```python
from build123d import *

# Parameters (mm, degrees)
F0_R     = 1.55
F1_DEPTH = 4
F2_R     = 3
F3_DEPTH = 3


with BuildPart() as f1:
    # F0 (on Top) → F1 (new body)
    with BuildSketch(Plane.XY):
        Polygon((25.166199, 37.371666), (-19.243801, 37.371666), (-19.243801, -14.908334), (-24.348801, -14.908334), (-24.348801, -32.808334), (30.271199, -32.808334), (30.271199, -6.428334), (25.166199, -6.428334), align=None)
        with Locations((-20.908801, -17.408334)):
            Circle(F0_R, mode=Mode.SUBTRACT)
        with Locations((27.351199, -18.678334)):
            Circle(F0_R, mode=Mode.SUBTRACT)
        with Locations((-6.183801, 33.401666)):
            Circle(F0_R, mode=Mode.SUBTRACT)
        with Locations((21.756199, 33.401666)):
            Circle(F0_R, mode=Mode.SUBTRACT)
    extrude(amount=F1_DEPTH)

    # F2 (on face) → F3 (cut)
    with BuildSketch(Plane.XY.offset(4)):
        with Locations((-20.908801, -17.408334)):
            Circle(F2_R)
        with Locations((27.452319, -18.754228)):
            Circle(F2_R)
        with Locations((-6.183801, 33.401666)):
            Circle(F2_R)
        with Locations((21.756199, 33.401666)):
            Circle(F2_R)
    extrude(amount=-F3_DEPTH, mode=Mode.SUBTRACT)


solid = f1.part
```
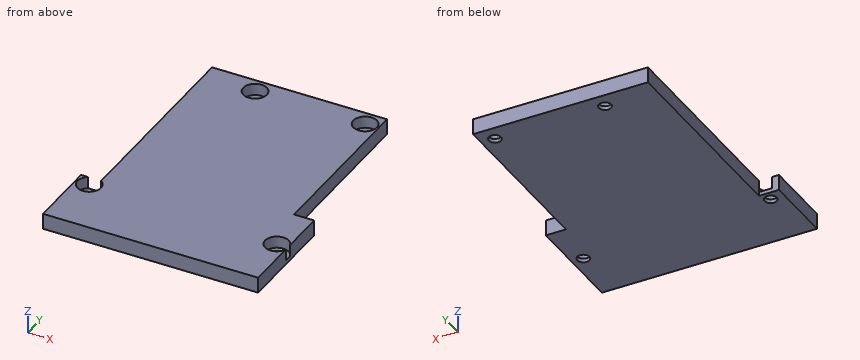
Work out the finished part from the listing and answer in its coordinate system (mm). Round coordinates to 2 decimals unless told otherwise and drop trailing zeros. Write each loop counter-clockwise with the first axis right and the second up, starting at its lowest first coordinate (ties: lowest second). Pieces come first, ordered by that corner, then holes.
1) A cutting plane is placed at B-B on z = 2.2. Give the number of separate pieces and of enclosed holes in the cut face, and give its area (3 significant figures).
2) Flat-ended cylindrical pins translate along their axes: P1, Ø1.2, axis at y = 19, z = 2.5, coming from the +X side; P2, Ø5.5, axis at x = 21.76, y = 33.4, coming from the -Z side; P3, Ø1.5, axis at y = 23, z = 1.5, coming from the -X side; P4, Ø1.8, axis at x = -5, y = 34.5, coming from the +Z side. Find the tip coordinate at first contact, or state that the pin passes through.
3) A cutting plane is placed at D-D on y = -9.5. Determine the outline of the cut face in (x, z).
4) Consider probe 1 along Y at (x, z) = (22, 3.85); probe 2 along X at (y, z) = (13, 0.5); probe 3 along Y at (x, z) = (27, 1.3). Determine where each line is inside the solid, lowest interval first.
5) A cutting plane is placed at C-C on y = 17.5. Determine the outline of the cut face in (x, z).
6) A cutting plane is placed at A-A on x = -21. Determine the outline of the cut face in (y, z), and give its area (3 significant figures).
Entries:
1. separate pieces: 1
1. enclosed holes: 2
1. area: 3,230 mm2
2. P1: stops at x = 25.17
2. P2: stops at z = 0
2. P3: stops at x = -19.24
2. P4: stops at z = 1
3. outline: (-19.24, 0) - (30.27, 0) - (30.27, 4) - (-19.24, 4) - close
4. probe 1: y = -32.81 to 30.41, 36.39 to 37.37
4. probe 2: x = -19.24 to 25.17
4. probe 3: y = -32.81 to -21.72, -15.79 to -6.43
5. outline: (-19.24, 0) - (25.17, 0) - (25.17, 4) - (-19.24, 4) - close
6. outline: (-32.81, 0) - (-18.96, 0) - (-18.96, 1) - (-20.41, 1) - (-20.41, 4) - (-32.81, 4) - close; (-15.86, 0) - (-14.91, 0) - (-14.91, 1) - (-15.86, 1) - close
6. area: 52.0 mm2
